Autodesk Inventor part; units mm, degrees
ref_plane "YZ Plane" through (0, 0, 0) normal (1, 0, 0) x (0, 1, 0)
ref_plane "XZ Plane" through (0, 0, 0) normal (0, 1, 0) x (-1, 0, 0)
ref_plane "XY Plane" through (0, 0, 0) normal (0, 0, 1) x (1, 0, 0)
sketch "Sketch1" plane through (0, 0, 0) normal (1, 0, 0) x (0, 1, 0)
  line L0 (-25, 25) -> (25, 25)
  line L1 (25, 25) -> (25, -25)
  line L2 (25, -25) -> (-25, -25)
  line L3 (-25, -25) -> (-25, 25)
  point P0 (0, 0)
  dimension "d0" = 50
  dimension "d1" = 50
  dimension "d2" = 25
  dimension "d3" = 25
extrude "Extrusion1" add sketch "Sketch1" along normal blind 6
sketch "Sketch2" plane through (6, 0, 0) normal (1, 0, 0) x (0, 0, -1)
  point P0 (0, 0)
  point P1 (0, 0)
hole "Hole1" at (6, 0, 0) direction (-1, 0, 0) diameter 12 end through all
fillet "Fillet2" radius 12 4 edges at (3, 25, 25) (3, 25, -25) (3, -25, -25) (3, -25, 25)
equation "\"d0\" = hoop_tabs_width"
equation "\"d1\" = hoop_tabs_width"
equation "\"d4\" = hoop_tabs_thickness"
equation "\"d6\" = hoop_tabs_hole"
equation "\"d14\" = hoop_tabs_hole"
equation "\"hoop_tabs_width\" = 50"
equation "\"hoop_tabs_thickness\" = 6"
equation "\"hoop_tabs_hole\" = 12"
equation "\"hoop_angle_z\" = 45deg"
equation "\"hoop_bearing_length\" = 5deg"
equation "\"hoop_cable_diam\" = 5"
equation "\"hoop_cable_pulley_diam\" = 22"
equation "\"hoop_thickness_large\" = 4"
equation "\"hoop_thickness_medium\" = 3.2"
equation "\"hoop_thickness_small\" = 2"
equation "\"hoop_width_large\" = 51"
equation "\"hoop_width_medium\" = 33.7"
equation "\"hoop_width_small\" = 25.4"
equation "\"rack_tooth_addendum\" = 5"
equation "\"rack_tooth_dedendum\" = 5"
equation "\"rack_tooth_thickness\" = 5"
equation "\"secure_arm_angle\" = 35deg"
equation "\"secure_arm_radii\" = 9"
equation "\"support_baseClamp_platformLengthBuffer\" = 35"
equation "\"support_baseClamp_platformThickness\" = 15"
equation "\"support_baseClamp_platformWidthBuffer\" = 0"
equation "\"support_baseClamp_sleeveHoleDiameter\" = 12"
equation "\"support_baseClamp_sleeveSweepTerminationAngle\" = 55deg"
equation "\"support_baseClamp_thickness\" = 8"
equation "\"support_frame_endHoleBuffer\" = 45"
equation "\"support_frame_squareBarFillet\" = 2"
equation "\"support_frame_squareBarThickness\" = 5"
equation "\"wheelchair_deployed_width\" = 635"
equation "\"wheelchair_deployed_length\" = 1067"
equation "\"wheelchair_deployed_height\" = 914"
equation "\"sm_varx_squareBarThickness\" = 2.5"
equation "\"sm_varx_pinPlate_thickness\" = 5"
equation "\"sm_varx_pinPlate_holeDiameter\" = 5"
equation "\"sm_varx_member_tolerance\" = 0"
equation "\"hoop_bushing12_radialInterference\" = 0"
equation "\"hoop_bushing23_radialInterference\" = 0"
equation "\"hoop_bushing23_od\" = -2 * hoop_thickness_medium + hoop_width_medium + hoop_bushing23_radialInterference"
equation "\"hoop_bushing12_od\" = -2 * hoop_thickness_large + hoop_width_large + hoop_bushing12_radialInterference"
equation "\"wheelchatir_pos_deploy_angle_0\" = 65deg"
equation "\"wheelchatir_pos_store_angle_0\" = 90deg"
equation "\"wheelchatir_pos_deploy_angle_1\" = 20deg"
equation "\"wheelchatir_pos_store_angle_1\" = 20deg"
equation "\"hoop_bushing12_thickness\" = -hoop_width_medium + hoop_bushing12_od - 2 * hoop_bushing12_radialInterference"
equation "\"hoop_bushing23_thickness\" = -hoop_width_small + hoop_bushing23_od - 2 * hoop_bushing23_radialInterference"
properties part number "hoop_tab" material "Steel, Mild"
Here's how the part is built. I have some questions about the finished solid (model axes, mm). Round coordinates to 2 decimals unless told otherwise and drop trailing zeros. Write each loop counter-clockwise with the first axis right and the second up, starting at its lowest first coordinate (ties: lowest second). Pieces come first, ordered by that corner, then holes.
1. If we mould it in two halves opening along Y, with no side actions, what happens to faces 1 (the flat face through (3, 25, 0)), 2 (the flat face through (3, -25, 0)), 3 (the flat face through (3, 0, -25)), 4 (the cylindrical face through (3, 0, 6))? For each: released by +Y, released by -Y, zero draft, split by the parting line, or undercut.
2. Suppose I cut it at C-C (x = 1.05). List the corners of the cut face in (y, z) for me, and give its area (3 significant figures).
3. I need wall thicknesses on L1, parallel to Y at x = 2.65, z = 0; L2, parallel to Y at x = 2.05, z = 4.5. Which ranges of each line are inside material? Lowest first, please.
4. Suppose I cut it at A-A (z = 0). List the corners of the cut face in (x, y) for me.
5. Suppose I cut it at D-D (y = 16). List the corners of the cut face in (x, z) for me.
6. Will this pin go through, and if not, where does the flat tip stop? pin 1 Ø7 at (y, z) = (0, 0) entering from -X.
Answer sheet:
1. face 1: released by +Y
1. face 2: released by -Y
1. face 3: zero draft
1. face 4: undercut
2. outline: (-25, -13) arc R12 ccw to (-13, -25) - (13, -25) arc R12 ccw to (25, -13) - (25, 13) arc R12 ccw to (13, 25) - (-13, 25) arc R12 ccw to (-25, 13) - close; hole circle Ø12 at (0, 0)
2. area: 2,260 mm2
3. L1: y = -25 to -6, 6 to 25
3. L2: y = -25 to -3.97, 3.97 to 25
4. outline: (0, -25) - (6, -25) - (6, -6) - (0, -6) - close; (0, 6) - (6, 6) - (6, 25) - (0, 25) - close
5. outline: (0, -24.62) - (6, -24.62) - (6, 24.62) - (0, 24.62) - close
6. pin 1: passes through
